Here's the drawing with two shaded views (mm, measured from the low corner). I have some questions. Give positions to 0.01 mm unless a question says otherwise; leave off trailing zeros. Loops run counter-clockwise (first coordinate to the right, second up) from the corner with the lowest first, then second, coordinate; pieces in that order, holes last. Notation, with made-up numbers: M -5,-29.75 L 5,-29.75 A20 ccw 5,-24.75 Z; hole C -17,61 d4. An arc over 180 degrees is marked long. Put each result on its own line as item: value. Start each with the question number.
1) Please list where these lines run through material, in increasing order: line 1 along Y through (x, z) = (47.5, 1) (1 decimal); line 2 along Y through (x, z) = (76.5, 1.8) (1 decimal). Write a range as from..to.
2) Imagine slicing it at C-C (x = 22). Write out the boundary of the cut face in (y, z) (1 decimal).
3) Imagine slicing it at B-B (z = 1.5). Write out the boundary of the cut face in (x, y) (1 decimal).
4) For P1, Ø2.5, axis at x = 76.5, y = 4.59, coming from the -Z side, with a flat end and sliding along its axis, tell me the tip position at first contact or that it passes through.
5) Imagine slicing it at A-A (x = 4.5). Write out the boundary of the cut face in (y, z) (1 decimal), then the cut area to 3 significant figures.
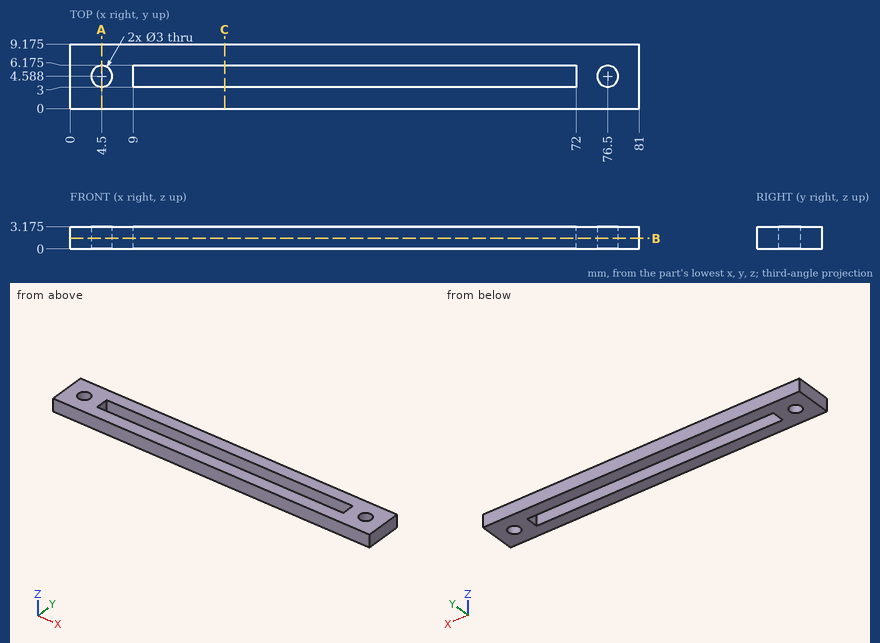
Recorded:
1. line 1: 0..3, 6.2..9.2
1. line 2: 0..3.1, 6.1..9.2
2. outline: M 0,0 L 3,0 L 3,3.2 L 0,3.2 Z; M 6.2,0 L 9.2,0 L 9.2,3.2 L 6.2,3.2 Z
3. outline: M 0,0 L 81,0 L 81,9.2 L 0,9.2 Z; hole C 4.5,4.6 d3; hole M 9,3 L 72,3 L 72,6.2 L 9,6.2 Z; hole C 76.5,4.6 d3
4. P1: through
5. outline: M 0,0 L 3.1,0 L 3.1,3.2 L 0,3.2 Z; M 6.1,0 L 9.2,0 L 9.2,3.2 L 6.1,3.2 Z
5. area: 19.6 mm²
